Autodesk Inventor part; units mm, degrees
ref_plane "YZ Plane" through (0, 0, 0) normal (1, 0, 0) x (0, 1, 0)
ref_plane "XZ Plane" through (0, 0, 0) normal (0, 1, 0) x (-1, 0, 0)
ref_plane "XY Plane" through (0, 0, 0) normal (0, 0, 1) x (1, 0, 0)
sketch "Sketch1" plane through (0, 0, 0) normal (0, 0, 1) x (1, 0, 0)
  line L0 (8.6603, -5) -> (0, -10)
  line L1 (0, -10) -> (-8.6603, -5)
  line L2 (-8.6603, -5) -> (-8.6603, 5)
  line L3 (-8.6603, 5) -> (0, 10)
  line L4 (0, 10) -> (8.6603, 5)
  line L5 (8.6603, 5) -> (8.6603, -5)
  point P0 (0, 0)
  point P1 (0, 0)
  dimension "d0" = 10
extrude "Extrusion1" add sketch "Sketch1" along normal blind 6
sketch "Sketch2" plane through (0, 0, 6) normal (0, 0, 1) x (1, 0, 0)
  circle A0 centre (0, 0) radius 8.6603
  line L0 (0, -10) -> (8.6603, -5)
extrude "Extrusion2" cut sketch "Sketch2" against normal blind 6 draft 45 keep common part
sketch "Sketch3" plane through (0, 0, 0) normal (0, 0, -1) x (-1, 0, 0)
  circle A0 centre (0, 0) radius 7.5
  dimension "d5" = 15
extrude "Extrusion3" add sketch "Sketch3" along normal blind 100
fillet "Fillet1" radius 1 1 edges at (7.5, 0, 0)
chamfer "Chamfer1" distance 1 angle 45 1 edges at (7.5, 0, -100)
sketch "Sketch4" plane through (0, 0, 0) normal (0, 1, 0) x (-1, 0, 0)
  point P0 (0, 0)
sketch "Sketch5" plane through (0, 0, 0) normal (0, 1, 0) x (-1, 0, 0)
  point P0 (0, 0)
thread "Thread1"
properties part number "Main Bolt"
Work out the finished part from the listing and answer in its coordinate system (mm). A direction names the side the tool comes from. Give positions to 0.01 mm unless a question says otherwise; leave off trailing zeros. Write each loop counter-clockwise with the first axis right and the second up, starting at its lowest first coordinate (ties: lowest second). Pieces come first, ordered by that corner, then holes.
Q1. The part is cut by section A-A on z = -3. Give the vertices of the cut face in (x, y), and give its area (3 significant figures).
Answer:
outline: circle Ø15 at (0, 0)
area: 177 mm2
Q2. A tool of negligible diameter and unlimited length cuts with its end or side. For faces 1 (the face through (-0.02, 8.99, 5.67)), 2 (the face through (7.493, -0.33, -49.314)), from which of +Z, -Z, +X, -X, +Y, -Y can it reach the whole face along a straight path? Write none if from no direction.
Answer:
face 1: +Z, +Y
face 2: -Z
Q3. Given pin 1 (3 mm diameter, centred on y = -4, z = -63.5, fed in from -X); pin 2 (5 mm diameter, centred on y = 3.5, z = -9, fed in from -X); pin 3 (5 mm diameter, centred on y = 0, z = -55, fed in from -X), each flat-ended and moving along its own axis, determine where each tip first touches the part or whether it passes through.
Answer:
pin 1: stops at x = -7.07
pin 2: stops at x = -7.43
pin 3: stops at x = -7.5
Q4. Straight lines are drawn through the part: L1, parallel to X at y = -3.75, z = -21.5; L2, parallel to Y at x = 1.5, z = -83.5; L3, parallel to X at y = -3.5, z = -90.5. For each, find the intervals that lie inside material, in ascending order.
Answer:
L1: x = -6.5 to 6.5
L2: y = -7.35 to 7.35
L3: x = -6.63 to 6.63
